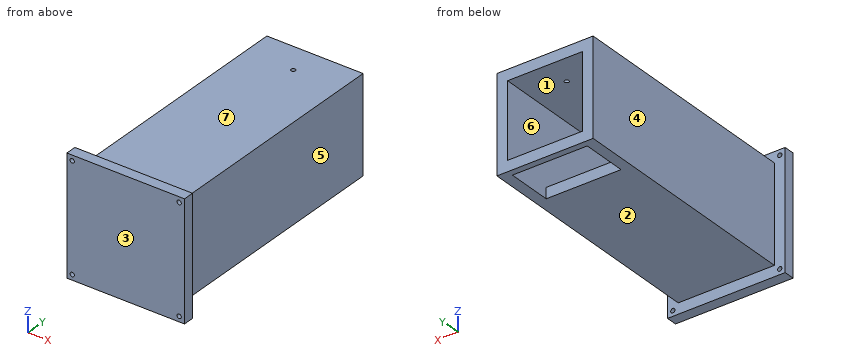
```python
from build123d import *

# Parameters (mm, degrees)
CROQUIS1_W                 = 45
CROQUIS1_H                 = 45
SALIENTE_EXTRUIR1_DEPTH    = 300
CROQUIS4_W                 = 18
CROQUIS4_H                 = 34
CORTAR_EXTRUIR2_DEPTH      = 46
CROQUIS8_W                 = 35
CROQUIS8_H                 = 35
CORTAR_EXTRUIR3_DEPTH      = 301
CROQUIS9_W                 = 35
CROQUIS9_H                 = 21.174410022
CORTAR_EXTRUIR4_DEPTH      = 10
CROQUIS10_R                = 1
CORTAR_EXTRUIR5_DEPTH      = 10
CROQUIS11_W                = 45
CROQUIS11_H                = 26.387879272
CORTAR_EXTRUIR6_DEPTH      = 46
CROQUIS13_W                = 45
CROQUIS13_H                = 160
CORTAR_EXTRUIR7_DEPTH      = 23.5
CORTAR_EXTRUIR7_DEPTH_BACK = 23.5
CROQUIS14_W                = 55
CROQUIS14_H                = 55
SALIENTE_EXTRUIR2_DEPTH    = 5
CROQUIS16_R                = 1
CORTAR_EXTRUIR8_DEPTH      = 1
CORTAR_EXTRUIR8_DEPTH_BACK = 119.612120728


with BuildPart() as part:
    # Croquis1 → Saliente-Extruir1 (new body)
    with BuildSketch(Plane(origin=(0, 0, 0), x_dir=(1, 0, 0), z_dir=(0, 1, 0))):
        Rectangle(CROQUIS1_W, CROQUIS1_H)
    extrude(amount=SALIENTE_EXTRUIR1_DEPTH)

    # Croquis4 → Cortar-Extruir2 (cut, through all)
    with BuildSketch(Plane.ZY.offset(22.5)):
        with Locations((13.5, 17)):
            Rectangle(CROQUIS4_W, CROQUIS4_H)
    extrude(amount=-CORTAR_EXTRUIR2_DEPTH, mode=Mode.SUBTRACT)

    # Croquis8 → Cortar-Extruir3 (cut, through all)
    with BuildSketch(Plane(origin=(0, 300, 0), x_dir=(1, 0, 0), z_dir=(0, 1, 0))):
        Rectangle(CROQUIS8_W, CROQUIS8_H)
    extrude(amount=-CORTAR_EXTRUIR3_DEPTH, mode=Mode.SUBTRACT)

    # Croquis9 → Cortar-Extruir4 (cut)
    with BuildSketch(Plane(origin=(0, 0, -22.5), x_dir=(-1, 0, 0), z_dir=(0, 0, -1))):
        with Locations((0, 260)):
            Rectangle(CROQUIS9_W, CROQUIS9_H)
    extrude(amount=-CORTAR_EXTRUIR4_DEPTH, mode=Mode.SUBTRACT)

    # Croquis10 → Cortar-Extruir5 (cut)
    with BuildSketch(Plane.XY.offset(22.5)):
        with Locations((0, 260)):
            Circle(CROQUIS10_R)
    extrude(amount=-CORTAR_EXTRUIR5_DEPTH, mode=Mode.SUBTRACT)

    # Croquis11 → Cortar-Extruir6 (cut, through all)
    with BuildSketch(Plane.XY.offset(22.5)):
        with Locations((0, 286.806060364)):
            Rectangle(CROQUIS11_W, CROQUIS11_H)
    extrude(amount=-CORTAR_EXTRUIR6_DEPTH, mode=Mode.SUBTRACT)

    # Croquis13 → Cortar-Extruir7 (cut, two sides)
    with BuildSketch(Plane(origin=(0, 0, 0), x_dir=(0, 0, -1), z_dir=(1, 0, 0))) as cortar_extruir7_sk:
        with Locations((0, 80)):
            Rectangle(CROQUIS13_W, CROQUIS13_H)
    extrude(amount=CORTAR_EXTRUIR7_DEPTH, mode=Mode.SUBTRACT)
    extrude(cortar_extruir7_sk.sketch, amount=-CORTAR_EXTRUIR7_DEPTH_BACK, mode=Mode.SUBTRACT)

    # Croquis14 → Saliente-Extruir2 (add)
    with BuildSketch(Plane.XZ.offset(-160)):
        Rectangle(CROQUIS14_W, CROQUIS14_H)
    extrude(amount=SALIENTE_EXTRUIR2_DEPTH)

    # Croquis16 → Cortar-Extruir8 (cut, two sides)
    with BuildSketch(Plane.XZ.offset(-155)) as cortar_extruir8_sk:
        with Locations((25, 25)):
            Circle(CROQUIS16_R)
        with Locations((-25, 25)):
            Circle(CROQUIS16_R)
        with Locations((-25, -25)):
            Circle(CROQUIS16_R)
        with Locations((25, -25)):
            Circle(CROQUIS16_R)
    extrude(amount=CORTAR_EXTRUIR8_DEPTH, mode=Mode.SUBTRACT)
    extrude(cortar_extruir8_sk.sketch, amount=-CORTAR_EXTRUIR8_DEPTH_BACK, mode=Mode.SUBTRACT)


solid = part.part
```
Design review of the part built by this model. Coordinates are the model's own, in mm. Face numbers are marked on the shaded views. A direction names the side the tool comes from. Coordinates: 2 decimals unless noted, no trailing zeros. Order: outer loops, then holes, each group sorted by start corner. A loop starts at its lowest first (then second) coordinate and runs counter-clockwise, first axis right, second up. Notation, with made-up numbers: M -2,74.5 L 52,74.5 A29 cw 52,103.5 Z; hole C 82,51.5 d4. An arc over 180 degrees is marked long. Answer as a JSON object with one key per item and string values. Group by question number.
1) Add section A-A, the plane y = 173. Write out the cut boundary in (x, z), then the cut area to 3 significant figures.
2) Add section C-C, the plane z = 21. Write out the cut boundary in (x, y), then the cut area to 3 significant figures.
3) For pin 1 (3 mm diameter, centred on x = -25, z = 25, fed in from +Y); pin 2 (2 mm diameter, centred on y = 209, z = -21.5, fed in from -X); pin 3 (17.5 mm diameter, centred on x = 8.5, y = 239, fed in from -Z), all flat-tipped, find the tip position at first contact; note any pin that passes through.
4) Tool access review of the marked faces 1, 2, 3 and 4: name each direction out of +Z, -Z, +X, -X, +Y, -Y from which nothing blocks a thin tool from reaching the whole face with its end or side.
5) Add section B-B, the plane x = 15. Write out the cut boundary in (y, z).
6) Wall thickness on L1, parallel to Z at x = -25, y = 156.45; L2, parallel to Z at x = 6.5, y = 176; L3, parallel to Y at x = 0, z = 19.95: over which ranges is each line inside the solid? List them lowest first.
7) Mouldability with a two-part tool opening along Z and no side actions: class the marked faces 5, 6 and 7 as pulls with the +Z half, pulls with the -Z half, needs draft (parallel to the pull), parting line crosses it, or undercut.
8) Add section D-D, the plane y = 257. Write out the cut boundary in (x, z).
Computed values:
{
 "1": {"outline": "M -22.5,-22.5 L 22.5,-22.5 L 22.5,22.5 L -22.5,22.5 Z; hole M -17.5,-17.5 L 17.5,-17.5 L 17.5,17.5 L -17.5,17.5 Z", "area": "800 mm^2"},
 "2": {"outline": "M -27.5,155 L 27.5,155 L 27.5,160 L 22.5,160 L 22.5,273.61 L -22.5,273.61 L -22.5,160 L -27.5,160 Z; hole C 0,260 d2", "area": "5,380 mm^2"},
 "3": {"pin 1": "stops at y = 160", "pin 2": "stops at x = -22.5", "pin 3": "stops at z = -22.5"},
 "4": {"face 1": "+Y", "face 2": "-Z, +X, -X, +Y", "face 3": "+Z, -Z, +X, -X, -Y", "face 4": "+Z, -Z, -X, +Y"},
 "5": {"outline": "M 155,-27.5 L 160,-27.5 L 160,-22.5 L 249.41,-22.5 L 249.41,-17.5 L 160,-17.5 L 160,17.5 L 273.61,17.5 L 273.61,22.5 L 160,22.5 L 160,27.5 L 155,27.5 Z; M 270.59,-22.5 L 273.61,-22.5 L 273.61,-17.5 L 270.59,-17.5 Z"},
 "6": {"L1": "z = -27.5 to -26, -24 to 24, 26 to 27.5", "L2": "z = -22.5 to -17.5, 17.5 to 22.5", "L3": "y = 155 to 259, 261 to 273.61"},
 "7": {"face 5": "needs draft", "face 6": "undercut", "face 7": "pulls with the +Z half"},
 "8": {"outline": "M -22.5,-22.5 L -17.5,-22.5 L -17.5,17.5 L 17.5,17.5 L 17.5,-22.5 L 22.5,-22.5 L 22.5,22.5 L -22.5,22.5 Z"}
}
